Here's how the part is built. I have some questions about the finished solid (model axes, mm). Face numbers are marked on the shaded views. A direction names the side the tool comes from. Coordinates: 2 decimals unless noted, no trailing zeros. Write each loop counter-clockwise with the first axis right and the second up, starting at its lowest first coordinate (ties: lowest second). Pieces come first, ordered by that corner, then holes. Notation, with made-up numbers: (46, 21) -> (89, 21) arc R3 ccw to (89, 26) -> close; hole circle Ø3 at (31, 40). An arc over 180 degrees is marked (long way). Use a Markdown table: item, result. Add a question column.
Item 1: If we mould it in two halves opening along Y, with no side actions, what happens to the marked faces 4, 5 and 6? For each: pulls with the +Y half, pulls with the -Y half, needs draft (parallel to the pull), parting line crosses it, or undercut.
Item 2: Imagine slicing it at C-C, the plane y = 40. Write out the boundary of the cut face in (x, z).
Item 3: On a 3-axis mill with a long thin cutter (end or side, diameter ignored), from which of +Z, -Z, +X, -X, +Y, -Y can I reach the whole of each face in a straight line? I mean the marked faces 1, 2 and 3. Say none if no direction works.
Item 4: If I drill on line 1 along X through (y, z) = (-12.45, -27.3); line 2 along Z through (x, y) = (-12, 30); line 3 along Y through (x, z) = (-19.75, -27.3), over which ranges is the centre line in solid material (lowest first)? Write a range as from..to.
Item 5: Imagine slicing it at B-B, the plane z = -43.25. Write out the boundary of the cut face in (x, y), and give its area (3 significant figures).
Item 6: Imagine slicing it at A-A, the plane x = 0. Write out the boundary of the cut face in (y, z).
Item 7: Will these pins go through, and if not, where does the flat tip stop? pin 1 Ø6 at (y, z) = (30, -27.3) entering from +X; pin 2 Ø5 at (x, y) = (22.5, 0) entering from +Z; pin 3 Ø3.5 at (y, z) = (30, -27.3) entering from -X; pin 4 Ø1 at (x, y) = (-10, 4.5) entering from +Z.
Item 8: Imagine slicing it at D-D, the plane x = -22.5. Write out the boundary of the cut face in (y, z), and give its area (3 significant figures).
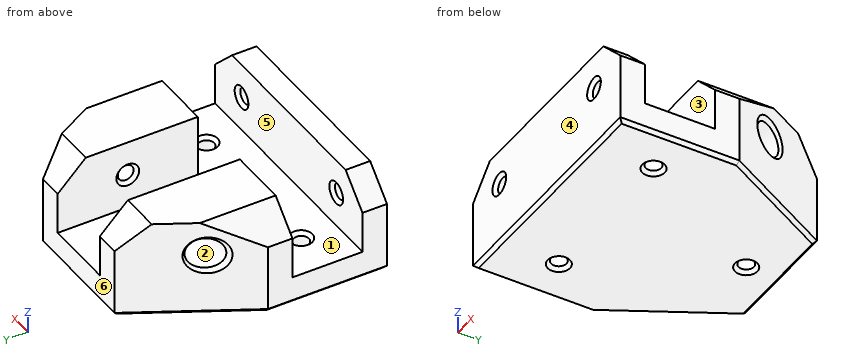
```python
from build123d import *

# Parameters (mm, degrees)
PAD014_DEPTH            = 28
POCKET008_DEPTH         = 20
SKETCH024_R             = 2.2
POCKET009_DEPTH         = 28.001
SKETCH025_R             = 2.25
POCKET010_DEPTH         = 17.001
SKETCH026_R             = 2.25
POCKET011_DEPTH         = 35.001
POCKET011_DEPTH_BACK    = 35.001
SKETCH027_R             = 4.5
POCKET012_DEPTH         = 219.723582
CHAMFER005_SIZE         = 8
CHAMFER006_SIZE         = 1
BODY008_PITCH_ANGLE     = 90
BODY008_PLACEMENT_ANGLE = -90


with BuildPart() as part:
    # Sketch022 → Pad014 (new body)
    with BuildSketch(Plane.YZ):
        Polygon((-35, 17), (-35, -17), (-17, -50), (17, -50), (35, -17), (35, 17), align=None)
    extrude(amount=PAD014_DEPTH)

    # Sketch023 → Pocket008 (cut)
    with BuildSketch(Plane.YZ):
        Polygon((-35, 10), (35, 10), (35, -10), (10, -10), (10, -50), (-10, -50), (-10, -10), (-35, -10), align=None)
    extrude(amount=POCKET008_DEPTH, mode=Mode.SUBTRACT)

    # Sketch024 → Pocket009 (cut, through all)
    with BuildSketch(Plane.YZ):
        with Locations((-22.5, 0)):
            Circle(SKETCH024_R)
        with Locations((22.5, 0)):
            Circle(SKETCH024_R)
        with Locations((0, -40)):
            Circle(SKETCH024_R)
    extrude(amount=POCKET009_DEPTH, mode=Mode.SUBTRACT)

    # Sketch025 → Pocket010 (cut, through all)
    with BuildSketch(Plane.XY):
        with Locations((10, 22.5)):
            Circle(SKETCH025_R)
        with Locations((10, -22.5)):
            Circle(SKETCH025_R)
    extrude(amount=POCKET010_DEPTH, mode=Mode.SUBTRACT)

    # Sketch026 → Pocket011 (cut, two sides)
    with BuildSketch(Plane.XZ) as pocket011_sk:
        with Locations((10, -30)):
            Circle(SKETCH026_R)
    extrude(amount=-POCKET011_DEPTH, mode=Mode.SUBTRACT)
    extrude(pocket011_sk.sketch, amount=POCKET011_DEPTH_BACK, mode=Mode.SUBTRACT)

    # Sketch027 (on Plane of DatumPlane) → Pocket012 (cut, through all)
    with BuildSketch(Plane.XZ.offset(-17)):
        with Locations((10, -30)):
            Circle(SKETCH027_R)
    pocket012 = extrude(amount=-POCKET012_DEPTH, mode=Mode.SUBTRACT)

    # Mirrored002: Pocket012 across XZ
    add(pocket012.mirror(Plane.XZ), mode=Mode.SUBTRACT)

    # Chamfer005
    chamfer005_edges = [part.edges().sort_by_distance(p)[0] for p in [
        (0, -35, 13.5),
        (0, 35, 13.5),
        (0, -13.5, -50),
        (0, 13.5, -50),
        (0, 35, -13.5),
        (0, -35, -13.5),
    ]]
    chamfer(chamfer005_edges, length=CHAMFER005_SIZE)

    # Chamfer006
    chamfer006_edges = [part.edges().sort_by_distance(p)[0] for p in [
        (28, -35, 0),
        (28, 0, 17),
        (28, -26, -33.5),
        (28, 35, 0),
        (28, 0, -50),
        (28, 26, -33.5),
        (28, 20.3, 0),
        (28, -2.2, -40),
        (28, -24.7, 0),
        (7.75, -22.5, 17),
        (7.75, 22.5, 17),
        (7.75, 22.5, 10),
        (7.75, -22.5, 10),
        (7.75, 10, -30),
        (7.75, -10, -30),
        (7.75, -17, -30),
        (7.75, 17, -30),
        (5.5, 27.909049, -30.000078),
        (5.5, -27.909133, -29.999922),
        (20, -2.2, -40),
        (20, 20.3, 0),
        (20, -24.7, 0),
    ]]
    chamfer(chamfer006_edges, length=CHAMFER006_SIZE)


with BuildPart() as part_1:
    # Body008 pitch: moved
    add(part.part.rotate(Axis((0, 0, 0), (0, 1, 0)), BODY008_PITCH_ANGLE))


with BuildPart() as part_2:
    # Body008 placement: moved
    add(part_1.part.moved(Location((0, 0, -17.3))).rotate(Axis((0, 0, -17.3), (0, 0, 1)), BODY008_PLACEMENT_ANGLE))


solid = part_2.part
```
Ans:
| question | item | result |
|---|---|---|
| 1 | face 4 | pulls with the -Y half |
| 1 | face 5 | undercut |
| 1 | face 6 | pulls with the +Y half |
| 2 | outline | (-22.45, -44.3) -> (-21.32, -45.3) -> (-3.2, -45.3) -> (-2.2, -44.3) -> (-2.2, -38.3) -> (-3.2, -37.3) -> (-10, -37.3) -> (-10, -17.3) -> (-22.45, -17.3) -> close; (2.2, -44.3) -> (3.2, -45.3) -> (21.32, -45.3) -> (22.45, -44.3) -> (22.45, -17.3) -> (10, -17.3) -> (10, -37.3) -> (3.2, -37.3) -> (2.2, -38.3) -> close |
| 3 | face 1 | +Z |
| 3 | face 2 | -X |
| 3 | face 3 | +Z, +X, -X |
| 4 | line 1 | x = -35..-24.75, -20.25..20.25, 24.75..35 |
| 4 | line 2 | z = -45.3..-29.55, -25.05..-17.3 |
| 4 | line 3 | y = -16.5..-10.5, 10..25.5, 34.5..44.96 |
| 5 | outline | (-35, -17) -> (35, -17) -> (35, 17) -> (17, 50) -> (-17, 50) -> (-35, 17) -> close; hole circle Ø4.4 at (-22.5, 0); hole circle Ø4.4 at (0, 40); hole circle Ø4.4 at (22.5, 0) |
| 5 | area | 4,050 mm^2 |
| 6 | outline | (-17, -44.3) -> (-16, -45.3) -> (36.8, -45.3) -> (37.8, -44.3) -> (37.8, -38.3) -> (36.8, -37.3) -> (-10, -37.3) -> (-10, -17.3) -> (-17, -17.3) -> close; (42.2, -44.3) -> (43.2, -45.3) -> (49, -45.3) -> (50, -44.3) -> (50, -37.3) -> (43.2, -37.3) -> (42.2, -38.3) -> close |
| 7 | pin 1 | stops at x = 16.75 |
| 7 | pin 2 | stops at z = -38 |
| 7 | pin 3 | passes through |
| 7 | pin 4 | stops at z = -37.3 |
| 8 | outline | (-17, -44.3) -> (-16, -45.3) -> (-3.2, -45.3) -> (-2.2, -44.3) -> (-2.2, -38.3) -> (-3.2, -37.3) -> (-10, -37.3) -> (-10, -30.55) -> (-11, -29.55) -> (-16, -29.55) -> (-17, -30.55) -> close; (-17, -24.05) -> (-16, -25.05) -> (-11, -25.05) -> (-10, -24.05) -> (-10, -17.3) -> (-17, -17.3) -> close; (2.2, -44.3) -> (3.2, -45.3) -> (37.83, -45.3) -> (39.92, -44.3) -> (39.92, -17.3) -> (10, -17.3) -> (10, -37.3) -> (3.2, -37.3) -> (2.2, -38.3) -> close; hole circle Ø9 at (30, -27.3) |
| 8 | area | 1,060 mm^2 |
